Autodesk Inventor part; units mm, degrees
ref_plane "YZ Plane" through (0, 0, 0) normal (1, 0, 0) x (0, 1, 0)
ref_plane "XZ Plane" through (0, 0, 0) normal (0, 1, 0) x (-1, 0, 0)
ref_plane "XY Plane" through (0, 0, 0) normal (0, 0, 1) x (1, 0, 0)
sketch "Sketch1" plane through (0, 0, 0) normal (0, 0, 1) x (1, 0, 0)
  line L0 (0, 0) -> (0, 8.6487)
  line L1 (0, 8.6487) -> (58.7375, 8.6487)
  line L2 (58.7375, 8.6487) -> (58.7375, 0)
  line L3 (58.7375, 0) -> (31.3531, 0)
  line L4 (31.3531, 0) -> (31.3531, 3.175)
  line L5 (31.3531, 3.175) -> (27.3844, 3.175)
  line L6 (27.3844, 3.175) -> (27.3844, 0)
  line L7 (27.3844, 0) -> (0, 0)
  dimension "d0" = 3.9688
  dimension "d1" = 3.175
  dimension "d2" = 58.7375
  dimension "d3" = 8.6487
extrude "Extrusion1" add sketch "Sketch1" against normal blind 4.7117
properties part number "VS-009 (SLIDE KEY)" material "Steel, Carbon"
Verification items for the finished model (mm, model axes). A direction names the side the tool comes from. Give positions to 0.01 mm unless a question says otherwise; leave off trailing zeros. Loops run counter-clockwise (first coordinate to the right, second up) from the corner with the lowest first, then second, coordinate; pieces in that order, holes last.
1. Section check C-C, the plane x = 30. Enter the section's corners in (y, z) (3 decimals), then the cut area to 3 significant figures.
2. Thickness scan on line 1 (X direction, y = 1.75, z = -0.15); line 2 (Y direction, x = 30, z = -3.25) (3 decimals). Record the ranges inside material, lowest first.
3. Section check A-A, the plane y = 1.25. Enter the section's corners in (x, z), then the cut area to 3 significant figures.
4. Mould release check, pull along X, two halves, no side actions. Record for faces 1 (the flat face through (14, 0, -2)), 2 (the flat face through (27.384, 2, -2)), 3 (the flat face through (0, 4, -2)): released by +X, released by -X, zero draft, split by the parting line, or undercut.
5. Section check B-B, the plane z = -2.55. Enter the section's corners in (x, y) (1 decimal).
6. Go/stop test with flat-tipped pins: pin 1 Ø5 at (x, y) = (48.5, 3) entering from +Z; pin 2 Ø2 at (x, z) = (29, -2.5) entering from -Y (3 decimals). Record where each tip stops, or that it passes through.
7. Set-up check for faces 4 (the flat face through (29, 8.649, -2)), 5 (the flat face through (29, 3.175, -2)): record each of +Z, -Z, +X, -X, +Y, -Y from which the full face is reachable in a straight line by a thin tool's end or side.
Geometry says:
1. outline: (3.175, -4.712) - (8.649, -4.712) - (8.649, 0) - (3.175, 0) - close
1. area: 25.8 mm2
2. line 1: x = 0 to 27.38, 31.35 to 58.74
2. line 2: y = 3.175 to 8.649
3. outline: (0, -4.71) - (27.38, -4.71) - (27.38, 0) - (0, 0) - close; (31.35, -4.71) - (58.74, -4.71) - (58.74, 0) - (31.35, 0) - close
3. area: 258 mm2
4. face 1: zero draft
4. face 2: undercut
4. face 3: released by -X
5. outline: (0, 0) - (27.4, 0) - (27.4, 3.2) - (31.4, 3.2) - (31.4, 0) - (58.7, 0) - (58.7, 8.6) - (0, 8.6) - close
6. pin 1: stops at z = 0
6. pin 2: stops at y = 3.175
7. face 4: +Z, -Z, +X, -X, +Y
7. face 5: +Z, -Z, -Y
